Check sheet for the drawn part. Datum: minimum x, y, z corner. Units: mm. A direction names the side the tool comes from. Give positions to 0.01 mm unless a question says otherwise; leave off trailing zeros. Order: outer loops, then holes, each group sorted by start corner. A loop starts at its lowest first (then second) coordinate and runs counter-clockwise, first axis right, second up. Notation, with made-up numbers: (60.5, -2) - (118.5, -2) arc R30 ccw to (118.5, 27) - close; hole circle Ø2 at (84.25, 21.5). An arc over 180 degrees is marked (long way). Answer as a JSON object with one key per item and string values. Group by question number.
(1) Section check B-B (z = 12.7). Count the separate pieces of the cut face and the enclosed holes in it, then the cut area to 3 significant figures.
(2) Section check A-A (x = 50.8). Record the boundary of the cut face in (y, z).
(3) Section check D-D (y = 8.75). Record the boundary of the cut face in (x, z).
(4) Mould release check, pull along X, two halves, no side actions. Record for the marked faces 1, 2, 3 and 4: +X half, -X half, draft (parallel to the pull), parting line (faces both ways), or undercut.
(5) Access from +Z, -Z, +X, -X, +Y, -Y to the whole of each face (thin tool, end or side, straight path). Record for the marked faces 5, 6 and 7.
(6) Thickness scan on line 1 (X direction, y = 3.5, z = 12.7); line 2 (Z direction, x = 50.8, y = 2); line 3 (X direction, y = 5.25, z = 11) (1 decimal). Record the ranges inside material, lowest first.
(7) Depth check by flat-ended pin: pin 1 Ø9 at (x, z) = (48.5, 14) entering from +Y (1 decimal); pin 2 Ø5.5 at (x, z) = (5, 9.5) entering from +Y; pin 3 Ø8 at (y, z) = (11, 22) entering from +X. Enter the tip coordinate at first touch or a pass-through.
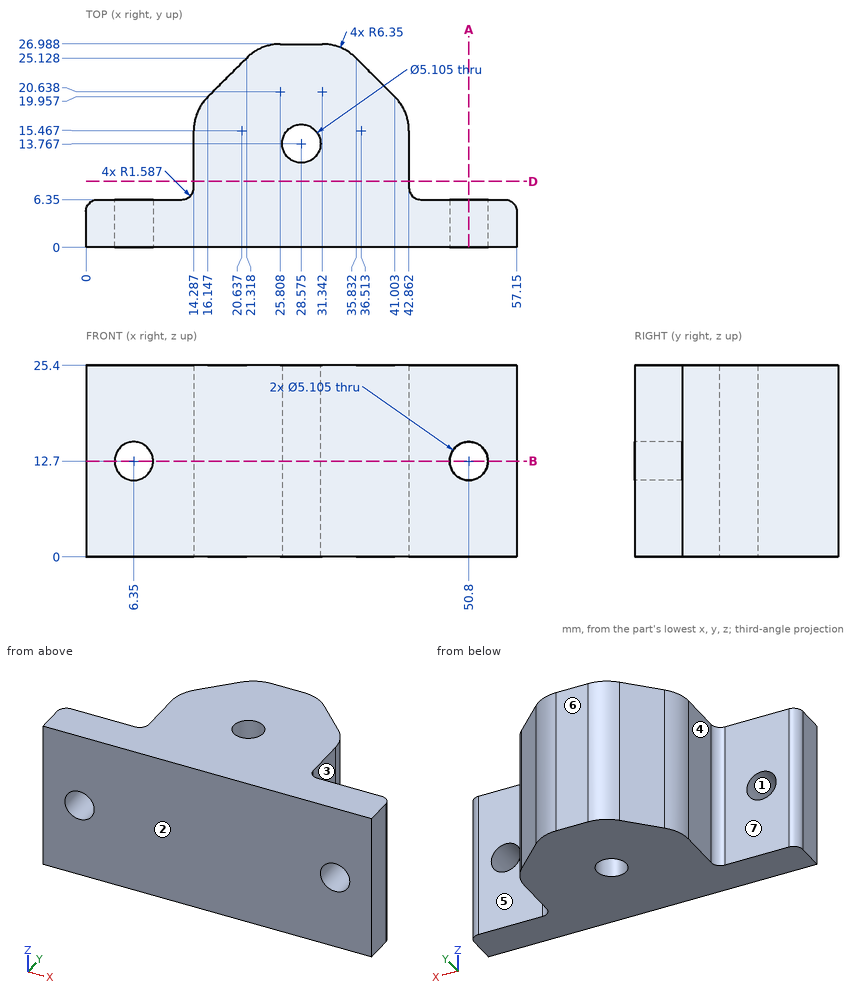
Solutions:
{
 "1": {"separate pieces": "3", "enclosed holes": "1", "area": "785 mm2"},
 "2": {"outline": "(0, 0) - (6.35, 0) - (6.35, 10.15) - (0, 10.15) - close; (0, 15.25) - (6.35, 15.25) - (6.35, 25.4) - (0, 25.4) - close"},
 "3": {"outline": "(14.29, 0) - (42.86, 0) - (42.86, 25.4) - (14.29, 25.4) - close"},
 "4": {"face 1": "undercut", "face 2": "draft", "face 3": "+X half", "face 4": "-X half"},
 "5": {"face 5": "+Z, -Z, +X, +Y", "face 6": "+Z, -Z, +X, -X, +Y", "face 7": "+Z, -Z, -X, +Y"},
 "6": {"line 1": "x = 0 to 3.8, 8.9 to 48.25, 53.35 to 57.15", "line 2": "z = 0 to 10.15, 15.25 to 25.4", "line 3": "x = 0.1 to 4.4, 8.3 to 48.9, 52.7 to 57.1"},
 "7": {"pin 1": "stops at y = 6.4", "pin 2": "stops at y = 6.35", "pin 3": "stops at x = 43.17"}
}
